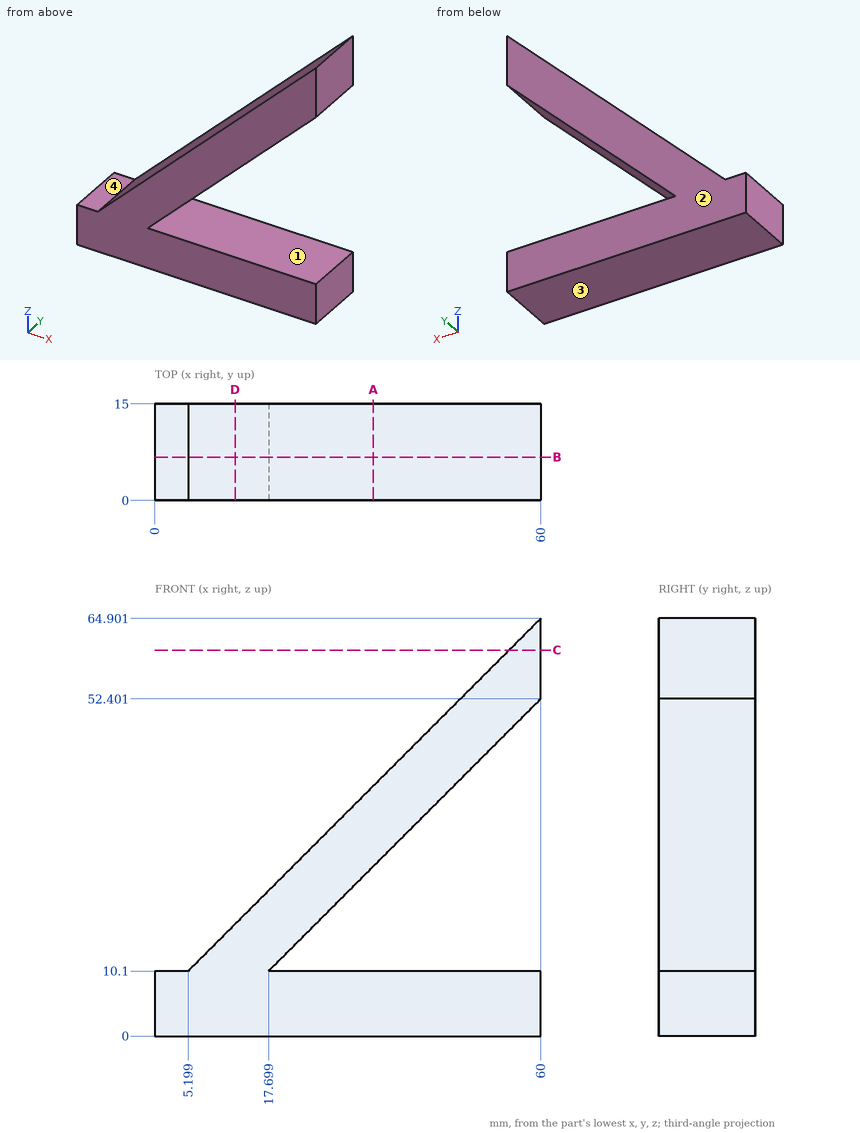
The figure shows three views and two pictorial views of one solid part (mm, origin at its lowest corner). Answer the questions. Round coordinates to 2 decimals unless told otherwise and drop trailing zeros. Write each loop counter-clockwise with the first axis right and the second up, starting at its lowest first coordinate (ties: lowest second). Pieces come first, ordered by that corner, then holes. Notation, with made-up numbers: (56.25, 23.5) -> (73.25, 23.5) arc R28 cw to (73.25, 56.5) -> close; hole circle Ø7 at (79.25, 81.25). An arc over 180 degrees is marked (long way). Answer as a JSON object with one key per item and string values. Group by question number.
Q1. Section C-C (z = 60) is taken. Write down the section's boundary in (x, y).
Q2. Determine the mould class of the marked faces 1, 2, 3 and 4 for opening direction Z: pulls with the +Z half, pulls with the -Z half, needs draft (parallel to the pull), parting line crosses it, or undercut.
Q3. Straight lines are drawn through the part: line 1 along Z through (x, y) = (29, 9.25); line 2 along Z through (x, y) = (43, 13); line 3 along Z through (x, y) = (9.5, 10). For each, find the intervals that lie inside material, in ascending order.
Q4. Each of these flat-tipped pins is pushed along its axis until it touches: pin 1 Ø6 at (y, z) = (7, 19) entering from +X; pin 2 Ø5 at (x, y) = (46.5, 12.5) entering from +Z; pin 3 Ø2 at (x, z) = (35.5, 11.5) entering from -Y; pin 4 Ø3 at (y, z) = (7.5, 40) entering from +X. Where does it stop, or does it pass through?
Q5. Section B-B (y = 6.75) is taken. Write down the section's boundary in (x, z).
Q6. Section D-D (x = 12.5) is taken. Write down the section's boundary in (y, z).
Q7. Section A-A (x = 34) is taken. Write down the section's boundary in (y, z).
Check values:
{
 "1": {"outline": "(55.1, 0) -> (60, 0) -> (60, 15) -> (55.1, 15) -> close"},
 "2": {"face 1": "undercut", "face 2": "needs draft", "face 3": "pulls with the -Z half", "face 4": "pulls with the +Z half"},
 "3": {"line 1": "0 to 10.1, 21.4 to 33.9", "line 2": "0 to 10.1, 35.4 to 47.9", "line 3": "0 to 14.4"},
 "4": {"pin 1": "x = 29.6", "pin 2": "z = 53.9", "pin 3": "through", "pin 4": "x = 49.1"},
 "5": {"outline": "(0, 0) -> (60, 0) -> (60, 10.1) -> (17.7, 10.1) -> (60, 52.4) -> (60, 64.9) -> (5.2, 10.1) -> (0, 10.1) -> close"},
 "6": {"outline": "(0, 0) -> (15, 0) -> (15, 17.4) -> (0, 17.4) -> close"},
 "7": {"outline": "(0, 0) -> (15, 0) -> (15, 10.1) -> (0, 10.1) -> close; (0, 26.4) -> (15, 26.4) -> (15, 38.9) -> (0, 38.9) -> close"}
}
